Autodesk Inventor part; units mm, degrees
ref_plane "MSC_PF1" through (0, 0, 0) normal (0, 1, 0) x (-1, 0, 0)
ref_plane "MSC_PT1" through (0, 0, -21.4001) normal (0, 0, -1) x (-1, 0, 0)
ref_plane "YZ Plane" through (0, 0, 0) normal (1, 0, 0) x (0, 1, 0)
sketch "Sketch2" plane through (0, 0, 0) normal (0, 1, 0) x (-1, 0, 0)
  line L0 (0, -21.4001) -> (0, -36.4001)
  line L1 (0, -36.4001) -> (5.125, -36.4001)
  line L2 (6, -35.5251) -> (6, -24.4001)
  line L3 (6, -24.4001) -> (5.35, -23.2742)
  line L4 (5.35, -23.2742) -> (5.35, -21.4001)
  line L5 (5.35, -21.4001) -> (0, -21.4001)
  line L6 (5.125, -36.4001) -> (6, -35.5251)
  line L7 (6, -36.4001) -> (6, -37.6375)
  line L8 (0, -40.885) -> (0, -18.1526)
  dimension "Ds" = 10.7
  dimension "NND" = 12
  dimension "b" = 12
  dimension "d3" = 30
  dimension "d5" = 45
  dimension "PTC" = 1.75
  dimension "NLG" = 15
revolve "Revolution1" add sketch "Sketch2" angle 360 about axis through (0, 0, -21.4001) along (0, 0, -1)
sketch "Sketch3" plane through (0, 0, -21.4001) normal (0, 0, 1) x (1, 0, 0)
  circle A0 centre (0, 0) radius 5.35
  line L0 (0, 9) -> (5.1962, 9)
  line L1 (5.1962, 9) -> (10.3923, 0)
  line L2 (10.3923, 0) -> (0, 0)
  line L3 (0, 0) -> (0, 9)
  line L4 (0, 9) -> (-5.1962, 9)
  line L5 (-5.1962, 9) -> (-10.3923, 0)
  line L6 (0, -9) -> (5.1962, -9)
  line L7 (5.1962, -9) -> (10.3923, 0)
  line L8 (-5.1962, -9) -> (-10.3923, 0)
  line L9 (0, -9) -> (-5.1962, -9)
  dimension "d9" = 60
  dimension "ParS" = 18
  dimension "msp_d11" = 18
extrude "Extrusion1" add sketch "Sketch3" along normal blind 7.5
sketch "Sketch4" plane through (0, 0, 0) normal (0, 1, 0) x (-1, 0, 0)
  line L0 (-9, -13.9001) -> (-10.3923, -13.9001)
  line L1 (-10.3923, -13.9001) -> (-10.3923, -14.7039)
  line L2 (-10.3923, -14.7039) -> (-9, -13.9001)
  line L3 (0, -25.2766) -> (0, 36.8591)
  line L4 (0, 27.9826) -> (0, 27.1787)
  line L5 (-10.3923, -21.4001) -> (-10.3923, -13.9001)
  line L6 (-5.1962, -13.9001) -> (-10.3923, -13.9001)
  dimension "d14" = 30
  dimension "msp_d15" = 18
revolve "Revolution2" cut sketch "Sketch4" angle 360 about axis through (0, 0, 27.9826) along (0, 0, -1)
sketch "Sketch5" plane through (0, 0, -13.9001) normal (0, 0, 1) x (1, 0, 0)
  arc A0 (7.7942, 4.5) -> (0, 9) centre (0, 0) ccw
  circle A1 centre (0, 0) radius 6.75
  dimension "d27" = 13.5
extrude "Extrusion2" cut sketch "Sketch5" against normal blind 1.5
thread "Thread1"
ref_plane "MSC_PF1" through (0, 0, 0) normal (0, 1, 0) x (-1, 0, 0)
ref_plane "MSC_PT1" through (0, 0, -21.4001) normal (0, 0, -1) x (-1, 0, 0)
fillet "Fillet1" radius 0.6 1 edges at (5.35, 0, -21.4001)
equation "\"msp_d11\" = ParS"
equation "\"msp_d15\" = ParS"
equation "\"d27\" = 0.75 * ParS"
equation "\"d28\" = 0.2 * ParK"
equation "\"d30\" = r"
equation "\"msp_d17\" = b"
equation "\"r\" = 0.6"
equation "\"THREADDIA\" = NND"
properties part number "ISO 4015 - M12 x 45" material "Stainless Steel, 440C"
Verification items for the finished model (mm, model axes). A direction names the side the tool comes from. Coordinates: 2 decimals unless noted, no trailing zeros. Order: outer loops, then holes, each group sorted by start corner. A loop starts at its lowest first (then second) coordinate and runs counter-clockwise, first axis right, second up. Notation, with made-up numbers: M -3,0.25 L 34,0.25 A26 cw 34,33.25 Z; hole C 79.5,51 d11. An arc over 180 degrees is marked long. One line per item, written item: value. Start each with the question number.
Item 1: Thickness scan on probe 1 along Y at (x, z) = (0, -14.3); probe 2 along Z at (x, y) = (-2.75, -4.25); probe 3 along Z at (x, y) = (6, -6.25). Record the ranges inside material, lowest first.
Item 2: Sectioned sample at B-B on z = -24. Record the cut outline in (x, y), then the cut area to 3 significant figures.
Item 3: Mould release check, pull along Y, two halves, no side actions. Record for faces 1 (the flat face through (0, 0, -36.4)), 2 (the cylindrical face through (-1.46, -6.59, -14.64)), 3 (the cylindrical face through (1.16, 5.223, -22.628)): pulls with the +Y half, pulls with the -Y half, needs draft (parallel to the pull), parting line crosses it, or undercut.
Item 4: Depth check by flat-ended pin: P1, Ø10, axis at x = -7, z = -19, coming from the -Y side; P2, Ø3, axis at y = 6, z = -33.5, coming from the -X side; P3, Ø4, axis at x = -2, z = -31, coming from the +Y side; P4, Ø6, axis at x = 5.5, z = -32, coming from the +Y side. Enter the tip coordinate at first touch or a pass-through.
Item 5: Sectioned sample at A-A on z = -17.5. Record the cut outline in (x, y), then the cut area to 3 significant figures.
Item 6: Access from +Z, -Z, +X, -X, +Y, -Y to the whole of each face (thin tool, end or side, straight path). Record for faces 4 (the flat face through (0, 0, -15.4)), 5 (the conical face through (-4.649, -8.099, -14.095)).
Calculated:
1. probe 1: -9 to -6.75, 6.75 to 9
1. probe 2: -36.4 to -15.4
1. probe 3: -21.4 to -13.9
2. outline: C 0,0 d11.54
2. area: 105 mm^2
3. face 1: needs draft
3. face 2: undercut
3. face 3: parting line crosses it
4. P1: y = -9
4. P2: x = -3.97
4. P3: y = 6
4. P4: y = 5.45
5. outline: M -10.39,0 L -5.2,-9 L 5.2,-9 L 10.39,0 L 5.2,9 L -5.2,9 Z
5. area: 281 mm^2
6. face 4: +Z
6. face 5: +Z, -X, -Y
